Autodesk Inventor part; units mm, degrees
ref_plane "YZ Plane" through (0, 0, 0) normal (1, 0, 0) x (0, 1, 0)
ref_plane "XZ Plane" through (0, 0, 0) normal (0, 1, 0) x (-1, 0, 0)
ref_plane "XY Plane" through (0, 0, 0) normal (0, 0, 1) x (1, 0, 0)
sketch "Sketch3" plane through (0, 0, 0) normal (0, 1, 0) x (-1, 0, 0)
  line L0 (-44, 50) -> (44, 50)
  line L1 (44, 50) -> (44, -50)
  line L2 (44, -50) -> (-44, -50)
  line L3 (-44, -50) -> (-44, 50)
  line L4 (-44, 50) -> (44, -50) construction
  line L5 (44, 50) -> (-44, -50) construction
  line L6 (44, 50) -> (-44, 50)
  line L7 (-44, 50) -> (-44, 47)
  line L8 (-44, 47) -> (44, 47)
  line L9 (44, 47) -> (44, 50)
  line L10 (44, 47) -> (41, 47)
  line L11 (41, 47) -> (41, -50)
  line L12 (41, -50) -> (44, -50)
  line L13 (44, -50) -> (44, 47)
  line L14 (-44, 47) -> (-41, 47)
  line L15 (-41, 47) -> (-41, -50)
  line L16 (-41, -50) -> (-44, -50)
  line L17 (-44, -50) -> (-44, 47)
  line L18 (41, -50) -> (-41, -50)
  line L19 (-41, -50) -> (-41, -47)
  line L20 (-41, -47) -> (41, -47)
  line L21 (41, -47) -> (41, -50)
  line L22 (41, 47) -> (34, 47)
  line L23 (34, 47) -> (34, -50)
  line L24 (34, -50) -> (37, -50)
  line L25 (37, -50) -> (37, 50)
  line L26 (34, 47) -> (34, 50)
  line L27 (41, 47) -> (41, 50)
  line L28 (-41, 47) -> (-41, 50)
  point P0 (0, 0)
  point P1 (37, -47)
  point P2 (37, 47)
  point P3 (34, -47)
  point P4 (37, 50)
  dimension "d33" = 88
  dimension "d34" = 100
  dimension "d35" = 88
  dimension "d36" = 3
  dimension "d37" = 3
  dimension "d38" = 3
  dimension "d39" = 3
  dimension "d63" = 7
  dimension "d64" = 3
extrude "Extrusion2" add sketch "Sketch3" along normal blind 100 contours L8 L15 L2 L3 | L8 L25 L20 L23 | L20 L23 L2 L15 | L20 L25 L2 L23
sketch "Sketch6" plane through (44, 0, -50) normal (0, 0, -1) x (-1, 0, 0)
  circle A0 centre (62.07, 7.54) radius 1.5875
  circle A1 centre (10, 12.62) radius 1.5875
  circle A2 centre (10, 40.56) radius 1.5875
  line L0 (7.46, 10.08) -> (7.46, 42.846)
  line L1 (7.46, 42.846) -> (10, 45.386)
  line L2 (10, 45.386) -> (10, 58.34)
  line L3 (10, 7.54) -> (7.46, 10.08)
  line L4 (10, 5) -> (10, 7.54)
  line L5 (76.04, 5) -> (10, 5)
  line L6 (76.04, 58.34) -> (76.04, 5)
  line L7 (10, 58.34) -> (76.04, 58.34)
  circle A3 centre (60.8, 55.8) radius 1.5875
  line L8 (0, 0) -> (81, 0)
  line L9 (0, 100) -> (81, 100)
  line L10 (0, 0) -> (0, 100)
  line L11 (0, 0) -> (0, 100)
  line L12 (0, 0) -> (10, 0)
  line L13 (78, 0) -> (3, 0)
  line L14 (10, 0) -> (10, 5)
  line L15 (81, 0) -> (81, 100)
  point P0 (44, 0)
  point P1 (85, 0)
  dimension "d52" = 10
  dimension "d53" = 5
  dimension "d54" = 90
extrude "Extrusion4" cut sketch "Sketch6" against normal up to surface (3 mm away) contours A0 | A1 | A2 | A3
sketch "Sketch9" plane through (-37, 0, -50) normal (-1, 0, 0) x (0, 0, 1)
  line L0 (17.33, 50.02) -> (31.33, 50.02)
  line L1 (31.33, 50.02) -> (31.33, 36.02)
  line L2 (31.33, 36.02) -> (17.33, 36.02)
  line L3 (17.33, 36.02) -> (17.33, 50.02)
  line L4 (17.65, 20.175) -> (32.65, 20.175)
  line L5 (32.65, 20.175) -> (32.65, 5.175)
  line L6 (32.65, 5.175) -> (17.65, 5.175)
  line L7 (17.65, 5.175) -> (17.65, 20.175)
  point P0 (50, 0)
extrude "Extrusion6" cut sketch "Sketch9" against normal up to surface (3 mm away)
sketch "Sketch10" plane through (44, 0, 50) normal (1, 0, 0) x (0, 0, -1)
  circle A0 centre (23.979, 79.591) radius 1.0922
  circle A1 centre (62.841, 79.591) radius 1.0922
  circle A2 centre (62.841, 54.191) radius 1.0922
  line L0 (21.82, 50) -> (21.82, 81.75)
  line L1 (65, 50) -> (21.82, 50)
  line L2 (65, 81.75) -> (65, 50)
  line L3 (21.82, 81.75) -> (65, 81.75)
  circle A3 centre (23.979, 54.191) radius 1.0922
  line L4 (3, 0) -> (100, 0)
  line L5 (100, 0) -> (100, 100)
  line L6 (3, 100) -> (100, 100)
  line L7 (100, 0) -> (100, 100)
  line L8 (100, 100) -> (65, 100)
  line L9 (3, 100) -> (100, 100)
  line L10 (100, 100) -> (135, 100) construction
  line L11 (100, 0) -> (100, 100)
  line L12 (65, 100) -> (65, 0)
  line L13 (100, 0) -> (3, 0)
  line L14 (3, 0) -> (3, 100)
  point P0 (50, 0)
  point P1 (0, 0)
  point P2 (0, 100)
  dimension "d67" = 35
  dimension "d68" = 180
  dimension "d75" = 100
extrude "Extrusion7" cut sketch "Sketch10" against normal up to surface (3 mm away) contours A0 | A1 | A2 | A3
sketch "Sketch11" plane through (-37, 0, -50) normal (-1, 0, 0) x (0, 0, 1)
  circle A0 centre (75.1, 71.8) radius 1.55
  circle A1 centre (75.1, 15.4) radius 1.55
  line L0 (67.45, 5) -> (82.75, 5)
  line L1 (67.45, 82.2) -> (82.75, 82.2)
  line L2 (95, 82.2) -> (95, 5)
  line L3 (55.2, 82.2) -> (55.2, 5)
  line L4 (32.65, 5.175) -> (17.65, 5.175)
  line L5 (17.65, 5.175) -> (17.65, 20.175)
  line L6 (17.65, 20.175) -> (32.65, 20.175)
  line L7 (32.65, 20.175) -> (32.65, 5.175)
  line L8 (31.33, 50.02) -> (31.33, 36.02)
  line L9 (31.33, 36.02) -> (17.33, 36.02)
  line L10 (17.33, 36.02) -> (17.33, 50.02)
  line L11 (17.33, 50.02) -> (31.33, 50.02)
  line L12 (0, 0) -> (97, 0)
  line L13 (0, 100) -> (97, 100)
  line L14 (0, 0) -> (0, 100)
  line L15 (100, 0) -> (100, 100)
  line L16 (100, 0) -> (100, 5)
  line L17 (100, 5) -> (95, 5)
  line L18 (97, 0) -> (97, 100)
  point P0 (50, 0)
  dimension "d71" = 5
  dimension "d72" = 5
extrude "Extrusion8" [suppressed]
sketch "Sketch12" plane through (-34, 0, -47) normal (0, 0, 1) x (1, 0, 0)
  circle A0 centre (17.2, 55.8) radius 1.5875
  circle A1 centre (68, 40.56) radius 1.5875
  circle A2 centre (15.93, 7.54) radius 1.5875
  circle A3 centre (68, 12.62) radius 1.5875
  line L0 (0, 0) -> (75, 0)
  line L1 (75, 0) -> (75, 100)
  line L2 (0, 100) -> (75, 100)
  line L3 (0, 0) -> (0, 100)
  line L4 (75, 0) -> (75, 100)
  line L5 (75, 100) -> (70, 100)
  line L6 (70, 100) -> (70, 70)
  line L7 (70, 70) -> (75, 70)
  line L8 (75, 70) -> (75, 100)
  point P0 (34, 0)
  dimension "d76" = 5
  dimension "d77" = 30
extrude "Extrusion9" add sketch "Sketch12" along normal blind 4.8 contours L7 L6 L2 L1
sketch "Sketch13" plane through (-34, 0, -42.2) normal (0, 0, 1) x (1, 0, 0)
  line L0 (70, 100) -> (70, 70)
  line L1 (70, 70) -> (75, 70)
  line L2 (75, 100) -> (75, 70)
  line L3 (75, 100) -> (70, 100)
  line L4 (70, 100) -> (70, 70)
  line L5 (75, 100) -> (70, 100)
  line L6 (70, 100) -> (70, 97)
  line L7 (70, 97) -> (75, 97)
  line L8 (75, 97) -> (75, 100)
  point P0 (34, 0)
  dimension "d80" = 3
extrude "Extrusion10" add sketch "Sketch13" along normal blind 2.4 contours L3 L2 L7 L0
sketch "Sketch14" plane through (-34, 0, -47) normal (0, 0, 1) x (1, 0, 0)
  line L0 (75, 0) -> (75, 70)
  line L1 (0, 0) -> (0, 100)
  line L2 (75, 0) -> (0, 0)
  line L3 (0, 0) -> (0, 3)
  line L4 (0, 3) -> (75, 3)
  line L5 (75, 3) -> (75, 0)
  point P0 (34, 0)
  dimension "d83" = 3
extrude "Extrusion11" add sketch "Sketch14" along normal up to surface (94 mm away)
sketch "Sketch15" plane through (-37, 0, 47) normal (0, 0, 1) x (1, 0, 0)
  line L0 (0, 0) -> (81, 0)
  line L1 (81, 0) -> (81, 100)
  line L2 (78, 100) -> (81, 100)
  line L3 (78, 3) -> (78, 100)
  line L4 (3, 3) -> (78, 3)
  line L5 (3, 3) -> (3, 100)
  line L6 (0, 100) -> (3, 100)
  line L7 (0, 0) -> (0, 100)
  point P0 (37, 0)
extrude "Extrusion12" add sketch "Sketch15" along normal blind 30
sketch "Sketch16" plane through (-37, 0, -50) normal (-1, 0, 0) x (0, 0, 1)
  line L0 (17.65, 5.175) -> (17.65, 20.175)
  line L1 (17.65, 20.175) -> (32.65, 20.175)
  line L2 (32.65, 20.175) -> (32.65, 5.175)
  line L3 (32.65, 5.175) -> (17.65, 5.175)
  line L4 (17.33, 50.02) -> (31.33, 50.02)
  line L5 (31.33, 50.02) -> (31.33, 36.02)
  line L6 (31.33, 36.02) -> (17.33, 36.02)
  line L7 (17.33, 36.02) -> (17.33, 50.02)
  line L8 (0, 0) -> (127, 0)
  line L9 (127, 100) -> (127, 0)
  line L10 (0, 100) -> (127, 100)
  line L11 (0, 0) -> (0, 100)
  circle A0 centre (75.1, 71.8) radius 1.55
  line L12 (75.1, 71.8) -> (75.1, 91.8)
  line L13 (75.1, 91.8) -> (83.1, 91.8)
  line L14 (75.1, 91.8) -> (67.1, 91.8)
  circle A1 centre (83.1, 91.8) radius 2
  circle A2 centre (67.1, 91.8) radius 2
  line L15 (127, 3) -> (127, 100)
  line L16 (127, 51.5) -> (71.1, 51.5)
  line L17 (75.1, 11.2) -> (83.1, 11.2)
  line L18 (75.1, 11.2) -> (67.1, 11.2)
  circle A3 centre (83.1, 11.2) radius 2
  circle A4 centre (67.1, 11.2) radius 2
  line L19 (83.1, 11.2) -> (91.1, 11.2)
  line L20 (67.1, 11.2) -> (59.1, 11.2)
  line L21 (127, 3) -> (3, 3)
  circle A5 centre (59.1, 11.2) radius 2
  circle A6 centre (91.1, 11.2) radius 2
  line L22 (91.1, 11.2) -> (99.1, 11.2)
  line L23 (99.1, 11.2) -> (99.1, 21.2)
  line L24 (99.1, 21.2) -> (51.1, 21.2)
  circle A7 centre (99.1, 21.2) radius 2
  circle A8 centre (51.1, 21.2) radius 2
  point P0 (50, 0)
  dimension "d88" = 20
  dimension "d89" = 8
  dimension "d90" = 8
  dimension "d91" = 4
  dimension "d92" = 4
  dimension "d95" = 8
  dimension "d96" = 8
  dimension "d97" = 4
  dimension "d98" = 4
  dimension "d99" = 8
  dimension "d100" = 10
  dimension "d101" = 48
  dimension "d102" = 4
  dimension "d103" = 4
extrude "Extrusion13" [suppressed]
sketch "Sketch17" plane through (44, 0, -50) normal (1, 0, 0) x (0, 0, -1)
  circle A0 centre (-37.159, 79.591) radius 1.0922
  circle A1 centre (-76.021, 54.191) radius 1.0922
  circle A2 centre (-37.159, 54.191) radius 1.0922
  circle A3 centre (-76.021, 79.591) radius 1.0922
  line L0 (0, 0) -> (-127, 0)
  line L1 (0, 0) -> (0, 100)
  line L2 (0, 100) -> (-127, 100)
  line L3 (-127, 0) -> (-127, 100)
  line L4 (-127, 0) -> (-127, 100)
  line L5 (-127, 50) -> (-107, 50)
  circle A4 centre (-107, 50) radius 5.5
  line L6 (0, 0) -> (-127, 0)
  line L7 (-63.5, 0) -> (-63.5, 20)
  circle A5 centre (-63.5, 20) radius 5.5
  line L8 (0, 0) -> (0, 100)
  line L9 (0, 50) -> (-20, 50.02)
  line L10 (-17.33, 50.02) -> (-31.33, 50.02)
  circle A6 centre (-20, 50.02) radius 5.5
  line L11 (-107, 50) -> (-107, 70)
  line L12 (-20, 50.02) -> (-20, 70.02)
  circle A7 centre (-107, 70) radius 5.5
  circle A8 centre (-20, 70.02) radius 5.5
  point P0 (-50, 0)
  dimension "d104" = 20
  dimension "d105" = 11
  dimension "d106" = 20
  dimension "d107" = 11
  dimension "d110" = 20
  dimension "d111" = 11
  dimension "d112" = 20
  dimension "d113" = 20
  dimension "d114" = 11
  dimension "d115" = 11
extrude "Extrusion14" cut sketch "Sketch17" against normal up to surface (3 mm away) contours A8 | A7 | A5
sketch "Sketch18" plane through (44, 0, -50) normal (0, 0, -1) x (-1, 0, 0)
  circle A0 centre (40.5, 15.4) radius 1.55
  circle A1 centre (40.5, 71.8) radius 1.55
  circle A2 centre (40.5, 71.8) radius 1.55
  line L0 (40.5, 71.8) -> (40.5, 91.8)
  line L1 (40.5, 91.8) -> (48.5, 91.8)
  line L2 (40.5, 91.8) -> (32.5, 91.8)
  circle A3 centre (48.5, 91.8) radius 2
  circle A4 centre (32.5, 91.8) radius 2
  circle A5 centre (32.5, 11.2) radius 2
  line L3 (40.5, 11.2) -> (32.5, 11.2)
  line L4 (40.5, 11.2) -> (48.5, 11.2)
  circle A6 centre (48.5, 11.2) radius 2
  line L5 (48.5, 11.2) -> (56.5, 11.2)
  line L6 (32.5, 11.2) -> (24.5, 11.2)
  circle A7 centre (24.5, 11.2) radius 2
  circle A8 centre (56.5, 11.2) radius 2
  line L7 (56.5, 11.2) -> (64.5, 11.2)
  line L8 (64.5, 11.2) -> (64.5, 21.2)
  line L9 (64.5, 21.2) -> (16.5, 21.2)
  circle A9 centre (64.5, 21.2) radius 2
  circle A10 centre (16.5, 21.2) radius 2
  line L10 (0, 0) -> (81, 0)
  line L11 (40.5, 0) -> (40.5, 11.2)
  point P0 (44, 0)
  dimension "d116" = 20
  dimension "d117" = 8
  dimension "d118" = 8
  dimension "d119" = 4
  dimension "d120" = 4
  dimension "d121" = 8
  dimension "d122" = 8
  dimension "d123" = 4
  dimension "d124" = 4
  dimension "d125" = 8
  dimension "d126" = 10
  dimension "d127" = 48
  dimension "d128" = 4
  dimension "d129" = 4
extrude "Extrusion15" cut sketch "Sketch18" against normal up to surface (3 mm away) contours A0 | A1 | A4 | A3 | A10 | A9 L9 L8 | L8 L9 A9
sketch "Sketch19" plane through (-34, 0, -39.8) normal (0, 0, 1) x (1, 0, 0)
  line L0 (70, 97) -> (70, 70)
  circle A0 centre (70, 97) radius 61.75
  circle A1 centre (17.2, 55.8) radius 1.5875
  line L1 (17.2, 55.8) -> (30.55, 55.8)
  line L2 (30.55, 55.8) -> (30.55, 49.4946)
  circle A2 centre (30.55, 49.4946) radius 1.55
  point P0 (34, 0)
  dimension "d132" = 123.5
  dimension "d133" = 13.35
  dimension "d134" = 3.1
extrude "Extrusion16" cut sketch "Sketch19" against normal blind 13.375 contours A2 A0 | A0 L2 A2 | A2 L2 A0
equation "\"BendRadius\" = Thickness"
equation "\"BendReliefWidth\" = Thickness"
equation "\"BendReliefDepth\" = 0.5 * Thickness"
equation "\"CornerReliefSize\" = 4 * Thickness"
equation "\"MinimumRemnant\" = 2 * Thickness"
equation "\"TransitionRadius\" = BendRadius"
equation "\"JacobiRadiusSize\" = Thickness"
equation "\"GapSize\" = Thickness"
properties part number "obudowa" material "ABS Plastic"
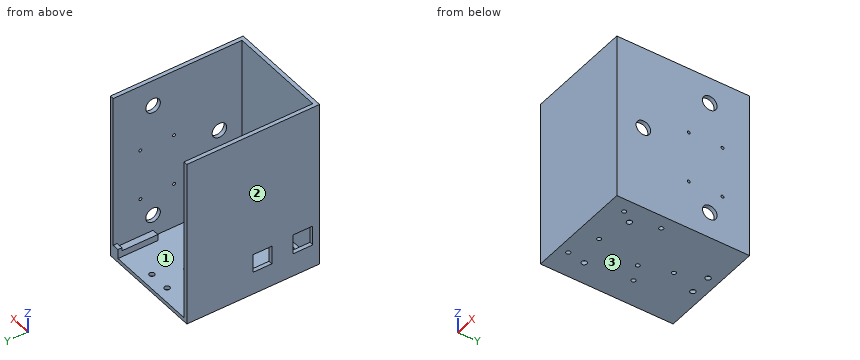
For this review, take the finished solid that the model builds, in its own axes (mm). Face numbers are marked on the shaded views. Coordinates: 2 decimals unless noted, no trailing zeros. Order: outer loops, then holes, each group sorted by start corner. A loop starts at its lowest first (then second) coordinate and runs counter-clockwise, first axis right, second up. Notation, with made-up numbers: (26, -24) -> (66, -24) arc R19 cw to (66, -6) -> close; hole circle Ø8 at (-34, 84). An arc over 180 degrees is marked (long way). Use CSV: the item, a comma, the result in double quotes. Start each with the question number.
Item 1: We need section C-C, the plane y = 7.54. Give the boundary of the cut face in (x, z), then the cut area to 3 significant figures.
Item 2: Wall thickness on probe 1 along X at (y, z) = (21, -48); probe 2 along Y at (x, z) = (3.5, -48.5); probe 3 along X at (y, z) = (40, 32): over which ranges is each line inside the solid? List them lowest first.
Item 3: We need section B-B, the plane z = -22. Give the boundary of the cut face in (x, y) (3 decimals), then the cut area to 3 significant figures.
Item 4: We need section D-D, the plane z = 13.5. Give the boundary of the cut face in (x, y).
Item 5: Insertion check: pin 1 (1.5 mm diameter, centred on x = -20.5, y = 53.5, fed in from +Z); pin 2 (3.5 mm diameter, centred on x = 38.5, y = 98, fed in from +Z); pin 3 (4 mm diameter, centred on x = 38.5, y = 79, fed in from +Z). Each pin has a flat end and moves straight along its axis. Give the tip position at first contact, or say it passes through.
Item 6: We need section A-A, the plane x = 34. Give the boundary of the cut face in (y, z), then the cut area to 3 significant figures.
Item 7: Draft analysis for pull direction X (two halves, no side actions). For the marked faces 1, 2 and 3, state which applies: pulls with the +X half, pulls with the -X half, needs draft (parallel to the pull), parting line crosses it, or undercut.
Derived:
1,outline,"(-37, -50) -> (-19.66, -50) -> (-19.66, -47) -> (-34, -47) -> (-34, -32.35) -> (-37, -32.35) -> close; (-37, -17.35) -> (-34, -17.35) -> (-34, 77) -> (-37, 77) -> close; (-16.48, -50) -> (44, -50) -> (44, 77) -> (41, 77) -> (41, -47) -> (-16.48, -47) -> close"
1,area,"932 mm^2"
2,probe 1,"x = -37 to -22.49, -18.51 to 25.51, 29.49 to 44"
2,probe 2,"y = 0 to 13.85, 16.95 to 70.25, 73.35 to 100"
2,probe 3,"x = -37 to -34, 41 to 44"
3,outline,"(-37, 0) -> (44, 0) -> (44, 100) -> (41, 100) -> (41, 3) -> (-34, 3) -> (-34, 5.175) -> (-37, 5.175) -> close; (-37, 20.175) -> (-34, 20.175) -> (-34, 36.02) -> (-37, 36.02) -> close; (-37, 50.02) -> (-34, 50.02) -> (-34, 100) -> (-37, 100) -> close"
3,area,"738 mm^2"
4,outline,"(-37, 0) -> (44, 0) -> (44, 14.5) -> (41, 14.5) -> (41, 3) -> (-34, 3) -> (-34, 100) -> (-37, 100) -> close; (41, 25.5) -> (44, 25.5) -> (44, 100) -> (41, 100) -> close"
5,pin 1,"stops at z = -47"
5,pin 2,"stops at z = -39.8"
5,pin 3,"stops at z = -42.2"
6,outline,"(0, -50) -> (11.03, -50) -> (11.03, -47) -> (3, -47) -> (3, 77) -> (0, 77) -> close; (14.21, -50) -> (38.97, -50) -> (38.97, -47) -> (14.21, -47) -> close; (42.15, -50) -> (100, -50) -> (100, -47) -> (42.15, -47) -> close"
6,area,"653 mm^2"
7,face 1,"undercut"
7,face 2,"pulls with the -X half"
7,face 3,"needs draft"
